from build123d import *

# Parameters (mm, degrees)
SKETCH_1_R               = 30
EXTRUDE_1_DEPTH          = 4
SKETCH_3_R               = 1.5
CUT_EXTRUDE_1_DEPTH      = 10
PATTERN_CIRCULAR_1_COUNT = 4
SKETCH_4_R               = 16
SKETCH_4_R_2             = 12.5
EXTRUDE_2_DEPTH          = 6


with BuildPart() as part:
    # 草图1 → 凸台-拉伸1 (new body)
    with BuildSketch(Plane.XY):
        Circle(SKETCH_1_R)
    extrude(amount=EXTRUDE_1_DEPTH)

    # 草图3 → 切除-拉伸1 (cut)
    with BuildSketch(Plane.XY.offset(4)):
        with Locations((0, 27)):
            Circle(SKETCH_3_R)
    cut_extrude_1 = extrude(amount=-CUT_EXTRUDE_1_DEPTH, mode=Mode.SUBTRACT)

    # 阵列(圆周)1: 切除-拉伸1 ×4 about axis
    pattern_circular_1_axis = Axis((0, 0, 0), (0, 0, 1))
    for i in range(1, PATTERN_CIRCULAR_1_COUNT):
        add(cut_extrude_1.rotate(pattern_circular_1_axis, i * 360 / PATTERN_CIRCULAR_1_COUNT), mode=Mode.SUBTRACT)

    # 草图4 → 凸台-拉伸2 (add)
    with BuildSketch(Plane(origin=(0, 0, 0), x_dir=(-1, 0, 0), z_dir=(0, 0, -1))):
        with Locations(Location((0, 0, 0), (0, 0, 180))):
            Circle(SKETCH_4_R)
        Circle(SKETCH_4_R_2, mode=Mode.SUBTRACT)
    extrude(amount=EXTRUDE_2_DEPTH)


solid = part.part
The model under review builds one solid part; all positions refer to its coordinate system, in mm. A direction names the side the tool comes from. Coordinates: 2 decimals unless noted, no trailing zeros. Loops run counter-clockwise (first coordinate to the right, second up) from the corner with the lowest first, then second, coordinate; pieces in that order, holes last. Notation, with made-up numbers: (-34, -28) -> (-13, -28) arc R13 ccw to (-13, -15) -> close; hole circle Ø5 at (18, -19). An arc over 180 degrees is marked (long way). Use a Markdown table: item, result. Add a question column.
1. Add section A-A on y = 0. Write out the cut boundary in (x, z).
2. To check wall thickness, follow line 1 (Y direction, x = 0, z = 1.6); line 2 (Z direction, x = 23.5, y = 14); line 3 (X direction, y = 3, z = -4). State the ranges of each line that lie inside material, in increasing order.
3. Clearance check with flat-ended pins moving along their axes: pin 1 Ø6 at (y, z) = (10, 2.5) entering from -X; pin 2 Ø6 at (y, z) = (11, -4) entering from -X; pin 3 Ø3 at (x, y) = (-1.5, 21.5) entering from -Z. State where each tip first meets the part, or that it passes through.
4. Add section D-D on x = -27. Write out the cut boundary in (y, z), plus the area to 3 significant figures.
5. Machinability: for faces 4 (the face through (-28.487, -0.195, 2.028)), 5 (the face through (-11.923, 3.755, -2.958)), which of the approach directions +Z, -Z, +X, -X, +Y, -Y give a long, thin tool a straight path to every point of the face, cutting with its end or side? Answer none if there is none.
6. Draft analysis for pull direction Y (two halves, no side actions). For faces 1 (the face through (28.487, 0.195, 2.028)), 2 (the face through (-29.97, 1.32, 1.97)), 3 (the face through (13, -13, 0)), state which applies: pulls with the +Y half, pulls with the -Y half, needs draft (parallel to the pull), parting line crosses it, or undercut.
7. Add section C-C on z = 1.75. Write out the cut boundary in (x, y), plus the area to 3 significant figures.
Returned:
| question | item | result |
|---|---|---|
| 1 | outline | (-30, 0) -> (-28.5, 0) -> (-28.5, 4) -> (-30, 4) -> close; (-25.5, 0) -> (-16, 0) -> (-16, -6) -> (-12.5, -6) -> (-12.5, 0) -> (12.5, 0) -> (12.5, -6) -> (16, -6) -> (16, 0) -> (25.5, 0) -> (25.5, 4) -> (-25.5, 4) -> close; (28.5, 0) -> (30, 0) -> (30, 4) -> (28.5, 4) -> close |
| 2 | line 1 | y = -30 to -28.5, -25.5 to 25.5, 28.5 to 30 |
| 2 | line 2 | z = 0 to 4 |
| 2 | line 3 | x = -15.72 to -12.13, 12.13 to 15.72 |
| 3 | pin 1 | stops at x = -29.17 |
| 3 | pin 2 | stops at x = -13.86 |
| 3 | pin 3 | stops at z = 0 |
| 4 | outline | (-13.08, 0) -> (-1.5, 0) -> (-1.5, 4) -> (-13.08, 4) -> close; (1.5, 0) -> (13.08, 0) -> (13.08, 4) -> (1.5, 4) -> close |
| 4 | area | 92.6 mm² |
| 5 | face 4 | +Z, -Z |
| 5 | face 5 | -Z |
| 6 | face 1 | undercut |
| 6 | face 2 | parting line crosses it |
| 6 | face 3 | needs draft |
| 7 | outline | circle Ø60 at (0, 0); hole circle Ø3 at (-27, 0); hole circle Ø3 at (0, -27); hole circle Ø3 at (0, 27); hole circle Ø3 at (27, 0) |
| 7 | area | 2,800 mm² |
